Input: part model. Units: mm. Frame: model coordinates. A direction names the side the tool comes from. Coordinates: 2 decimals unless noted, no trailing zeros. Loops run counter-clockwise (first coordinate to the right, second up) from the corner with the lowest first, then second, coordinate; pieces in that order, holes last. Notation, with made-up numbers: (78, 46) -> (114, 46) arc R26 ccw to (114, 71) -> close; hole circle Ø3 at (3, -24). An arc over 180 degrees is marked (long way). Put each result on its own line as item: value. Start each with the question number.
1) Cut plane A-A (x = 0). Return the cut outline in (y, z) (3 decimals).
2) Cut plane C-C (y = 8.75). State how many separate pieces and enclosed holes the cut face has, plus the area to 3 significant figures.
3) Pull-direction query (X, two-part tool) for faces 1 (the flat face through (67.289, 9.658, -67.415)), 2 (the cylindrical face through (20.91, 12.61, -10.66)), 3 (the flat face through (-1, 19.05, 20)); classes: pulls with the +X half, pulls with the -X half, needs draft (parallel to the pull), parting line crosses it, or undercut.
4) Cut plane B-B (z = 0). Return the cut outline in (x, y) (3 decimals), plus the area to 3 significant figures.
5) Contact query for flat-ended pins moving along their axis: P1, Ø6, axis at x = 50, y = 11, coming from the +Z side; P2, Ø3, axis at x = 46.5, y = 13.5, coming from the +Z side; P3, Ø6, axis at y = 17, z = 60, coming from the +X side. Output: stop coordinate, or through.
6) Set-up query: faces 4 (the flat face through (-29.383, 9.569, 80.532)), 5 (the flat face through (-58.31, 9.66, 67.29)). Return all of +Z, -Z, +X, -X, +Y, -Y with unobstructed straight access to the full face (end or side cutting, diameter ignored); none if empty.
7) Material intervals for L1, parallel to X at y = 2, z = 61; L2, parallel to Z at x = 53, y = 4.75; L3, parallel to X at y = 10.5, z = -84, sorted ascending.
from build123d import *

# Parameters (mm, degrees)
SKETCH1_R           = 98.425
BOSS_EXTRUDE1_DEPTH = 19.05
SKETCH3_R           = 3.5941
CUT_EXTRUDE4_DEPTH  = 19.05
CIRPATTERN2_COUNT   = 8
CUT_EXTRUDE5_DEPTH  = 12.7
CUT_EXTRUDE7_DEPTH  = 19.05
CIRPATTERN4_COUNT   = 4
SKETCH5_R           = 3.175
CUT_EXTRUDE8_DEPTH  = 12.7
CIRPATTERN5_COUNT   = 8
FILLET1_R           = 7.62


with BuildPart() as part:
    # Sketch1 → Boss-Extrude1 (new body)
    with BuildSketch(Plane(origin=(0, 0, 0), x_dir=(1, 0, 0), z_dir=(0, 1, 0))):
        Circle(SKETCH1_R)
    extrude(amount=BOSS_EXTRUDE1_DEPTH)

    # Sketch3 → Cut-Extrude4 (cut)
    with BuildSketch(Plane(origin=(0, 19.05, 0), x_dir=(1, 0, 0), z_dir=(0, 1, 0))):
        with Locations((-22.866976578, 53.758699595)):
            Circle(SKETCH3_R)
    cut_extrude4 = extrude(amount=-CUT_EXTRUDE4_DEPTH, mode=Mode.SUBTRACT)

    # CirPattern2: Cut-Extrude4 ×8 about axis
    cirpattern2_axis = Axis((0, 0, 0), (0, 1, 0))
    for i in range(1, CIRPATTERN2_COUNT):
        add(cut_extrude4.rotate(cirpattern2_axis, i * 360 / CIRPATTERN2_COUNT), mode=Mode.SUBTRACT)

    # Sketch4 → Cut-Extrude5 (cut)
    with BuildSketch(Plane(origin=(0, 19.05, 0), x_dir=(1, 0, 0), z_dir=(0, 1, 0))):
        with BuildLine():
            Line((-97.568819348, 12.954), (23.081180652, 12.954))
            Line((23.081180652, 12.954), (23.081180652, -12.954))
            Line((23.081180652, -12.954), (-97.568819348, -12.954))
            ThreePointArc((-97.568819348, -12.954), (-98.425, 0), (-97.568819348, 12.954))
        make_face()
    extrude(amount=-CUT_EXTRUDE5_DEPTH, mode=Mode.SUBTRACT)

    # Sketch2 → Cut-Extrude7 (cut)
    with BuildSketch(Plane(origin=(0, 19.05, 0), x_dir=(1, 0, 0), z_dir=(0, 1, 0))):
        Polygon((53.881536726, 62.861792847), (62.861792847, 71.842048969), (71.842048969, 62.861792847), (62.861792847, 53.881536726), align=None)
    cut_extrude7 = extrude(amount=-CUT_EXTRUDE7_DEPTH, mode=Mode.SUBTRACT)

    # CirPattern4: Cut-Extrude7 ×4 about axis
    cirpattern4_axis = Axis((0, 0, 0), (0, 1, 0))
    for i in range(1, CIRPATTERN4_COUNT):
        add(cut_extrude7.rotate(cirpattern4_axis, i * 360 / CIRPATTERN4_COUNT), mode=Mode.SUBTRACT)

    # Sketch5 → Cut-Extrude8 (cut)
    with BuildSketch(Plane(origin=(-33.663332607, 0, 92.489246201), x_dir=(0, -1, 0), z_dir=(-0.342020143, 0, 0.939692621))):
        with Locations((-9.525, -0.112232827)):
            Circle(SKETCH5_R)
    cut_extrude8 = extrude(amount=-CUT_EXTRUDE8_DEPTH, mode=Mode.SUBTRACT)

    # CirPattern5: Cut-Extrude8 ×8 about axis
    cirpattern5_axis = Axis((0, 0, 0), (0, 1, 0))
    for i in range(1, CIRPATTERN5_COUNT):
        add(cut_extrude8.rotate(cirpattern5_axis, i * 360 / CIRPATTERN5_COUNT), mode=Mode.SUBTRACT)

    # Fillet1
    fillet1_edges = [part.edges().sort_by_distance(p)[0] for p in [
        (23.081180652, 12.7, -12.954),
        (23.081180652, 12.7, 12.954),
    ]]
    fillet(fillet1_edges, radius=FILLET1_R)


solid = part.part
Results found:
1. outline: (0, -98.425) -> (19.05, -98.425) -> (19.05, -12.954) -> (6.35, -12.954) -> (6.35, 12.954) -> (19.05, 12.954) -> (19.05, 98.425) -> (0, 98.425) -> close
2. separate pieces: 1
2. enclosed holes: 12
2. area: 25,700 mm2
3. face 1: undercut
3. face 2: pulls with the -X half
3. face 3: needs draft
4. outline: (-98.425, 0) -> (98.425, 0) -> (98.425, 19.05) -> (23.081, 19.05) -> (23.081, 6.35) -> (-98.425, 6.35) -> close
4. area: 2,210 mm2
5. P1: stops at z = 86.48
5. P2: stops at z = 87.54
5. P3: stops at x = 80.24
6. face 4: none
6. face 5: +Y, -Y
7. L1: x = -77.24 to -69.98, -55.74 to 55.74, 69.98 to 77.24
7. L2: z = -82.94 to -26.38, -19.35 to 18.45, 25.24 to 82.94
7. L3: x = -51.3 to -42.38, -35.71 to 27.48, 33.91 to 51.3
